```python
from build123d import *

# Parameters (mm, degrees)
SKETCH1_R                = 45
BOSS_EXTRUDE1_DEPTH      = 15
CUT_EXTRUDE1_DEPTH       = 91.081591488
CUT_EXTRUDE1_DEPTH_BACK  = 91.081591488
M6_CLEARANCE_HOLE1_D     = 6.6
M6_CLEARANCE_HOLE1_DEPTH = 6
M6_CLEARANCE_HOLE1_TIP   = 1.982840043
M6_CLEARANCE_HOLE2_D     = 6.6
M6_CLEARANCE_HOLE2_DEPTH = 6
M6_CLEARANCE_HOLE2_TIP   = 1.982840043
M3_CLEARANCE_HOLE1_D     = 3.4
CIRPATTERN1_COUNT        = 6
CUT_EXTRUDE2_DEPTH       = 2


with BuildPart() as part:
    # Sketch1 → Boss-Extrude1 (new, symmetric)
    with BuildSketch(Plane.XY):
        with BuildLine():
            Line((-66.175, -15), (-66.175, 15))
            ThreePointArc((-66.175, 15), (-54.605786302, 18.103041727), (-46.142284003, 26.579167161))
            ThreePointArc((-46.142284003, 26.579167161), (0, 53.25), (46.142284003, 26.579167161))
            ThreePointArc((46.142284003, 26.579167161), (54.605786302, 18.103041727), (66.175, 15))
            Line((66.175, 15), (66.175, -15))
            ThreePointArc((66.175, -15), (54.605786302, -18.103041727), (46.142284003, -26.579167161))
            ThreePointArc((46.142284003, -26.579167161), (0, -53.25), (-46.142284003, -26.579167161))
            ThreePointArc((-46.142284003, -26.579167161), (-54.605786302, -18.103041727), (-66.175, -15))
        make_face()
        Circle(SKETCH1_R, mode=Mode.SUBTRACT)
    extrude(amount=BOSS_EXTRUDE1_DEPTH, both=True)

    # Sketch2 → Cut-Extrude1 (cut, two sides: drawn at the far end of the back side and taken through both)
    with BuildSketch(Plane.XY.offset(15).offset(-CUT_EXTRUDE1_DEPTH_BACK)):
        with BuildLine():
            Line((-60.175, -9.624867567), (-60.175, 9.624867567))
            ThreePointArc((-60.175, 9.624867567), (-55.795757401, 10.912645684), (-51.671575635, 12.868984861))
            ThreePointArc((-51.671575635, 12.868984861), (-53.25, 0), (-51.671575635, -12.868984861))
            ThreePointArc((-51.671575635, -12.868984861), (-55.795757401, -10.912645684), (-60.175, -9.624867567))
        make_face()
        with BuildLine():
            Line((60.175, -9.624867567), (60.175, 9.624867567))
            ThreePointArc((60.175, 9.624867567), (55.795757401, 10.912645684), (51.671575635, 12.868984861))
            ThreePointArc((51.671575635, 12.868984861), (53.25, 0), (51.671575635, -12.868984861))
            ThreePointArc((51.671575635, -12.868984861), (55.795757401, -10.912645684), (60.175, -9.624867567))
        make_face()
    extrude(amount=CUT_EXTRUDE1_DEPTH + CUT_EXTRUDE1_DEPTH_BACK, mode=Mode.SUBTRACT)

    # M6 Clearance Hole1
    with Locations(Plane.ZY.offset(66.175)):
        with Locations((0, 0)):
            Hole(M6_CLEARANCE_HOLE1_D / 2, depth=M6_CLEARANCE_HOLE1_DEPTH)
            with Locations((0, 0, -(M6_CLEARANCE_HOLE1_DEPTH + M6_CLEARANCE_HOLE1_TIP / 2))):  # 118° drill point
                Cone(0, M6_CLEARANCE_HOLE1_D / 2, M6_CLEARANCE_HOLE1_TIP, mode=Mode.SUBTRACT)

    # M6 Clearance Hole2
    with Locations(Plane(origin=(66.175, 0, 0), x_dir=(0, 0, -1), z_dir=(1, 0, 0))):
        with Locations((0, 0)):
            Hole(M6_CLEARANCE_HOLE2_D / 2, depth=M6_CLEARANCE_HOLE2_DEPTH)
            with Locations((0, 0, -(M6_CLEARANCE_HOLE2_DEPTH + M6_CLEARANCE_HOLE2_TIP / 2))):  # 118° drill point
                Cone(0, M6_CLEARANCE_HOLE2_D / 2, M6_CLEARANCE_HOLE2_TIP, mode=Mode.SUBTRACT)

    # M3 Clearance Hole1 (through all)
    with Locations(Plane.XY.offset(15)):
        with Locations((0, 49.125)):
            m3_clearance_hole1 = Hole(M3_CLEARANCE_HOLE1_D / 2)

    # CirPattern1: M3 Clearance Hole1 ×6 about axis
    cirpattern1_axis = Axis((0, 0, 0), (0, 0, 1))
    for i in range(1, CIRPATTERN1_COUNT):
        add(m3_clearance_hole1.rotate(cirpattern1_axis, i * 360 / CIRPATTERN1_COUNT), mode=Mode.SUBTRACT)

    # Sketch9 → Cut-Extrude2 (cut)
    with BuildSketch(Plane(origin=(-60.175, 0, 0), x_dir=(0, 0, -1), z_dir=(1, 0, 0))):
        Polygon((0, 5.888972746), (-5.1, 2.944486373), (-5.1, -2.944486373), (0, -5.888972746), (5.1, -2.944486373), (5.1, 2.944486373), align=None)
    cut_extrude2 = extrude(amount=-CUT_EXTRUDE2_DEPTH, mode=Mode.SUBTRACT)

    # Mirror1: Cut-Extrude2 across plane
    add(cut_extrude2.mirror(Plane(origin=(0, 0, 0), x_dir=(0, 0, 1), z_dir=(1, 0, 0))), mode=Mode.SUBTRACT)


solid = part.part
```
Build history of the part. All positions in model axes, mm. A direction names the side the tool comes from. Round coordinates to 2 decimals unless told otherwise and drop trailing zeros. Order: outer loops, then holes, each group sorted by start corner. A loop starts at its lowest first (then second) coordinate and runs counter-clockwise, first axis right, second up. Notation, with made-up numbers: (27.5, 41.5) -> (81.5, 41.5) arc R17 ccw to (81.5, 58.5) -> close; hole circle Ø3 at (-4.75, 68). An arc over 180 degrees is marked (long way). Answer in a Markdown table with one row per item.
1) Pin check, flat tips, straight feed: P1, Ø3, axis at x = 4, z = -5.5, coming from the -Y side; P2, Ø2, axis at x = 0, y = -49.125, coming from the -Z side; P3, Ø10, axis at x = 43, z = -1, coming from the -Y side; P4, Ø10, axis at x = -46.5, z = -8, coming from the -Y side. Stop position of each tip, or through.
Values:
| item | result |
|---|---|
| P1 | y = -53.19 |
| P2 | through |
| P3 | y = -37.3 |
| P4 | y = -33.37 |
2) Mould opens along Z. For faces 1 (the cylindrical face through (-0.369, -47.465, -0.21)), 2 (the flat face through (15, -43, -15)), 3 (the flat face through (-61.161, 4.396, -2.586)) say: released by +Z, released by -Z, zero draft, split by the parting line, or undercut.
Values:
| item | result |
|---|---|
| face 1 | zero draft |
| face 2 | released by -Z |
| face 3 | undercut |
3) Which spindle directions (+Z, -Z, +X, -X, +Y, -Y) get a long thin tool onto all of the face, cutting with end or side? Do faces 4 (the flat face through (-61.16, -4.44, -2.51)), 5 (the flat face through (-60.175, -4.4, 3.1)), 6 (the cylindrical face through (64.15, 2.23, -2.43)). Say none if no direction does.
Values:
| item | result |
|---|---|
| face 4 | none |
| face 5 | +Z, -Z |
| face 6 | +X |
4) Band-saw the part on C-C on y = -31. Give the cut face in (x, z), and give its area (3 significant figures).
Values:
| item | result |
|---|---|
| outline | (-43.3, -15) -> (-32.62, -15) -> (-32.62, 15) -> (-43.3, 15) -> close; (32.62, -15) -> (43.3, -15) -> (43.3, 15) -> (32.62, 15) -> close |
| area | 641 mm2 |
5) Band-saw the part on B-B on y = 0. Give the number of separate pieces and of enclosed holes in the cut face, and give its area (3 significant figures).
Values:
| item | result |
|---|---|
| separate pieces | 6 |
| enclosed holes | 0 |
| area | 761 mm2 |
6) Wall check: L1, parallel to X at y = 1, z = -12.5 (3 decimals); L2, parallel to X at y = -4, z = -2.5 (3 decimals); L3, parallel to Y at x = -16.5, z = 11.75. Give the ranges that are in metal, low to high.
Values:
| item | result |
|---|---|
| L1 | -66.175 to -60.175, -53.241 to -44.989, 44.989 to 53.241, 60.175 to 66.175 |
| L2 | -66.175 to -62.175, -53.1 to -44.822, 44.822 to 53.1, 62.175 to 66.175 |
| L3 | -50.63 to -41.87, 41.87 to 50.63 |
7) Band-saw the part on D-D on x = 18.5. Give the cut face in (y, z).
Values:
| item | result |
|---|---|
| outline | (-49.93, -15) -> (-41.02, -15) -> (-41.02, 15) -> (-49.93, 15) -> close; (41.02, -15) -> (49.93, -15) -> (49.93, 15) -> (41.02, 15) -> close |
8) Band-saw the part on A-A on x = 0. Give the cut face in (y, z) (3 decimals), and give its area (3 significant figures).
Values:
| item | result |
|---|---|
| outline | (-53.25, -15) -> (-50.825, -15) -> (-50.825, 15) -> (-53.25, 15) -> close; (-47.425, -15) -> (-45, -15) -> (-45, 15) -> (-47.425, 15) -> close; (45, -15) -> (47.425, -15) -> (47.425, 15) -> (45, 15) -> close; (50.825, -15) -> (53.25, -15) -> (53.25, 15) -> (50.825, 15) -> close |
| area | 291 mm2 |
